Here's the drawing with two shaded views (mm, measured from the low corner). I have some questions. Round coordinates to 2 decimals unless told otherwise and drop trailing zeros. Loops run counter-clockwise (first coordinate to the right, second up) from the corner with the lowest first, then second, coordinate; pieces in that order, holes last. Notation, with made-up numbers: M -18,7 L 40,7 A37 ccw 40,46 Z; hole C -12.75,83 d5. An arc over 180 degrees is marked long. Answer as a JSON object with one key per item and string values.
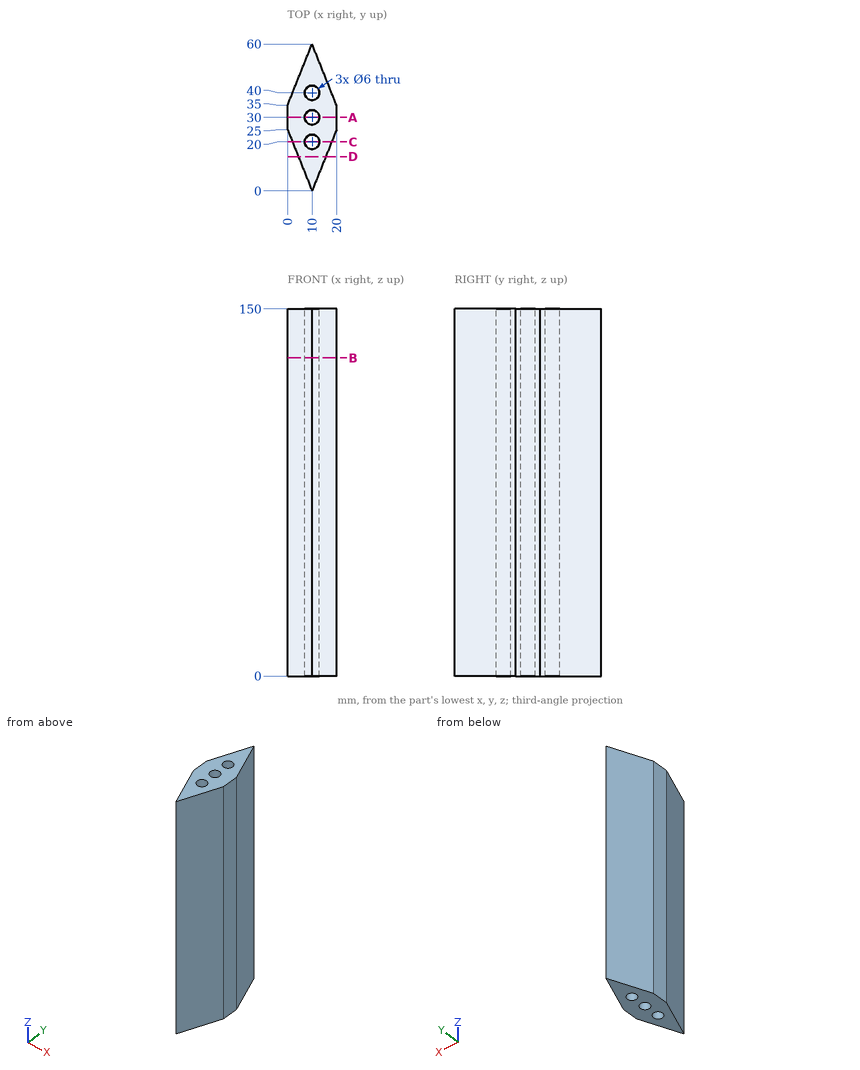
Item 1: If I drill on L1, parallel to X at y = 30, z = 69; L2, parallel to X at y = 20, z = 49; L3, parallel to X at y = 44, z = 71, over which ranges is the centre line in solid material (lowest first)? Write a range as from..to.
Solution:
{"L1": "x = 0..7, 13..20", "L2": "x = 2..7, 13..18", "L3": "x = 3.6..16.4"}
Item 2: I want a section at B-B on z = 130. Count the separate pieces of the cut face and the enclosed holes in it, plus the area to 3 significant figures.
Solution:
{"separate pieces": "1", "enclosed holes": "3", "area": "615 mm2"}
Item 3: I want a section at D-D on y = 14. List the corners of the cut face in (x, z) for me.
Solution:
{"outline": "M 4.4,0 L 15.6,0 L 15.6,150 L 4.4,150 Z"}
Item 4: For P1, Ø10, axis at x = 14, z = 52.5, coming from the +Y side; P2, Ø6, axis at y = 12, z = 27, coming from the +X side; P3, Ø3, axis at y = 12, z = 126.5, coming from the -X side, each with a flat end and sliding along its axis, tell me the tip position at first contact or that it passes through.
Solution:
{"P1": "stops at y = 60", "P2": "stops at x = 16", "P3": "stops at x = 4.6"}
Item 5: I want a section at A-A on y = 30. List the corners of the cut face in (x, z) for me.
Solution:
{"outline": "M 0,0 L 7,0 L 7,150 L 0,150 Z; M 13,0 L 20,0 L 20,150 L 13,150 Z"}
Item 6: I want a section at C-C on y = 20. List the corners of the cut face in (x, z) for me, plus the area to 3 significant figures.
Solution:
{"outline": "M 2,0 L 7,0 L 7,150 L 2,150 Z; M 13,0 L 18,0 L 18,150 L 13,150 Z", "area": "1,500 mm2"}
